Design review of the part shown in the three views and the two pictorial views. Dimensions are in mm from the part's minimum x, y and z. Round coordinates to 2 decimals unless told otherwise and drop trailing zeros. Loops run counter-clockwise (first coordinate to the right, second up) from the corner with the lowest first, then second, coordinate; pieces in that order, holes last. Notation, with made-up numbers: M -15.5,-33.5 L 32.5,-33.5 A23 cw 32.5,-4.5 Z; hole C 20,-15 d4. An arc over 180 degrees is marked long. One line per question, with ' | ' between items. Start each with the question number.
1) For probe 1 along Y at (x, z) = (97, 2.75); probe 2 along X at (y, z) = (43.5, 2.75) (1 decimal); probe 3 along X at (y, z) = (68.5, 1.5), list the stretches that pass through material, from the lowest coordinate up. Write a range as from..to.
2) For pin 1 Ø6 at (x, z) = (32, 8) entering from +Y; pin 2 Ø1.5 at (y, z) = (92, 4.5) entering from +X; pin 3 Ø1.5 at (y, z) = (25, 2) entering from +X; pin 4 Ø8 at (x, y) = (107.5, 102.5) entering from -Z, all flat-tipped, find the tip position at first contact; note any pin that passes through.
3) We need section A-A (x = 62). Give the boundary of the cut face in (y, z), and give its area (3 significant figures).
4) We need section C-C (y = 96). Give the boundary of the cut face in (x, z) (1 decimal).
5) We need section B-B (z = 2.5). Give the boundary of the cut face in (x, y) (1 decimal).
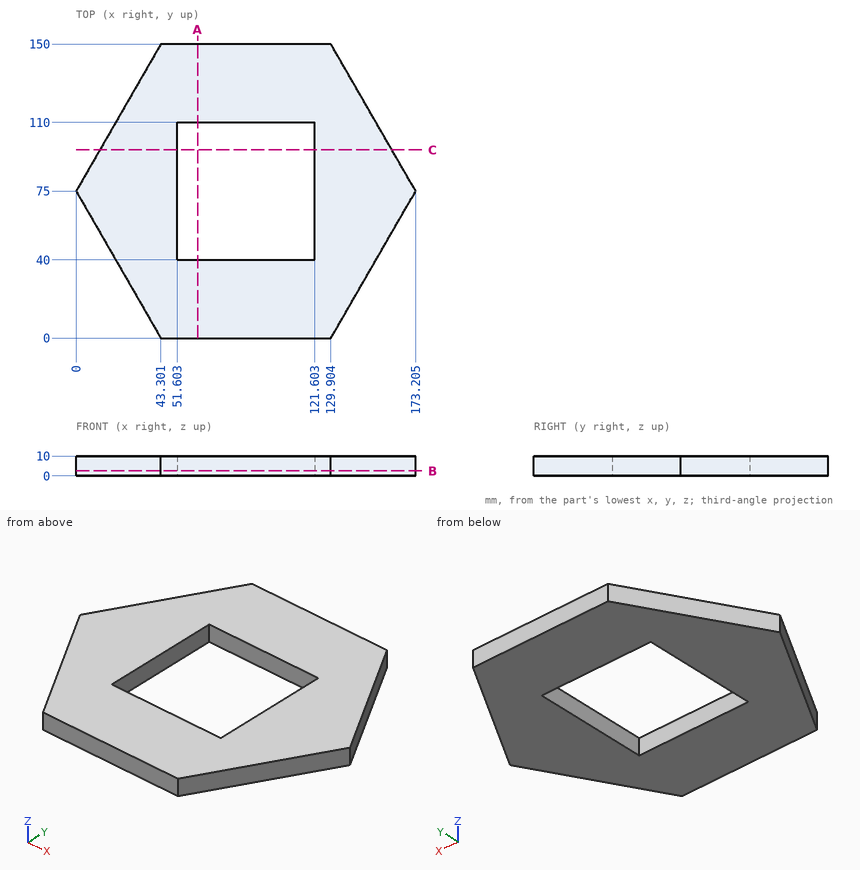
Answers below:
1) probe 1: 0..40, 110..150 | probe 2: 18.2..51.6, 121.6..155 | probe 3: 3.75..51.6, 121.6..169.45
2) pin 1: y = 135.62 | pin 2: x = 163.82 | pin 3: x = 144.77 | pin 4: through
3) outline: M 0,0 L 40,0 L 40,10 L 0,10 Z; M 110,0 L 150,0 L 150,10 L 110,10 Z | area: 800 mm^2
4) outline: M 12.1,0 L 51.6,0 L 51.6,10 L 12.1,10 Z; M 121.6,0 L 161.1,0 L 161.1,10 L 121.6,10 Z
5) outline: M 0,75 L 43.3,0 L 129.9,0 L 173.2,75 L 129.9,150 L 43.3,150 Z; hole M 51.6,40 L 121.6,40 L 121.6,110 L 51.6,110 Z
